from build123d import *

# Parameters (mm, degrees)
F1_DEPTH = 63.5
F2_DEPTH = 12.7
F3_R     = 5.08


with BuildPart() as f1:
    # F0 (on Front) → F1 (new body, symmetric)
    with BuildSketch(Plane.XZ):
        Polygon((19.77428763, 13.4614007547), (-32.80030936, 13.4614007547), (-32.80030936, -13.4614007547), (32.80030936, -13.4614007547), (32.80030936, 13.4614007547), align=None)
    extrude(amount=F1_DEPTH, both=True)

    # F0 (on Front) → F2 (join, symmetric)
    with BuildSketch(Plane.XZ):
        with BuildLine():
            Line((19.77428763, 24.8372294009), (19.77428763, 13.4614007547))
            Line((19.77428763, 13.4614007547), (32.80030936, 13.4614007547))
            Line((32.80030936, 13.4614007547), (32.80030936, 24.8372294009))
            ThreePointArc((32.80030936, 24.8372294009), (36.3320089212, 33.5525140508), (44.9345260859, 37.3506434262))
            Line((44.9345260859, 37.3506434262), (50.2432473004, 37.5140286498))
            Line((50.2432473004, 37.5140286498), (50.2432473004, 50.5462181007))
            Line((50.2432473004, 50.5462181007), (44.533817111, 50.3705003543))
            ThreePointArc((44.533817111, 50.3705003543), (26.9806216999, 42.6205237084), (19.77428763, 24.8372294009))
        make_face()
        Polygon((59.8447506625, 37.809531787), (50.2432473004, 37.5140286498), (50.2432473004, 33.1795029342), (59.9276782147, 33.1795029342), align=None)
        Polygon((59.5269692399, 55.5519722402), (59.8447506625, 37.809531787), (59.9276782147, 33.1795029342), (68.8237734139, 33.1795029342), (68.8237734139, 55.5519722402), align=None)
        Polygon((50.2432473004, 55.5519722402), (50.2432473004, 50.5462181007), (50.2432473004, 37.5140286498), (59.8447506625, 37.809531787), (59.5269692399, 55.5519722402), align=None)
    extrude(amount=F2_DEPTH, both=True)

    # F3
    f3_edges = [f1.edges().sort_by_distance(p)[0] for p in [
        (0, -63.5, 13.461401),
        (-32.800309, -63.5, 0),
        (0, -63.5, -13.461401),
        (32.800309, -63.5, 0),
        (-32.800309, 63.5, 0),
        (0, 63.5, -13.461401),
        (32.800309, 63.5, 0),
        (0, 63.5, 13.461401),
    ]]
    fillet(f3_edges, radius=F3_R)


solid = f1.part
For this review, take the finished solid that the model builds, in its own axes (mm). A direction names the side the tool comes from. Round coordinates to 2 decimals unless told otherwise and drop trailing zeros. Loops run counter-clockwise (first coordinate to the right, second up) from the corner with the lowest first, then second, coordinate; pieces in that order, holes last. Notation, with made-up numbers: (87, 78.5) - (121, 78.5) arc R34 cw to (121, 113.5) - close; hole circle Ø11 at (51, 14). An arc over 180 degrees is marked (long way). Use one line per item in the form item = value.
1) Wall thickness on probe 1 along Z at (x, y) = (15.5, 39); probe 2 along X at (y, z) = (12.5, 21); probe 3 along Z at (x, y) = (52, -8.5): over which ranges is each line inside the solid? List them lowest first.
Solutions:
probe_1 = -13.46 to 13.46
probe_2 = 19.77 to 32.8
probe_3 = 33.18 to 55.55
2) We need section C-C on z = -0.5. Write out the cut boundary in (x, y), then the cut area to 3 significant figures.
Solutions:
outline = (-32.8, -58.42) arc R5.08 ccw to (-27.72, -63.5) - (27.72, -63.5) arc R5.08 ccw to (32.8, -58.42) - (32.8, 58.42) arc R5.08 ccw to (27.72, 63.5) - (-27.72, 63.5) arc R5.08 ccw to (-32.8, 58.42) - close
area = 8,310 mm2
3) Mouldability with a two-part tool opening along X and no side actions: class faces 3 (the face through (0, -1, 13.461)), 4 (the face through (19.774, 0, 19)), 5 (the face through (36.239, -0.178, 33.455)) as pulls with the +X half, pulls with the -X half, needs draft (parallel to the pull), parting line crosses it, or undercut.
Solutions:
face_3 = needs draft
face_4 = pulls with the -X half
face_5 = undercut
4) We need section B-B on y = 5.5. Write out the cut boundary in (x, z), then the cut area to 3 significant figures.
Solutions:
outline = (-32.8, -13.46) - (32.8, -13.46) - (32.8, 24.84) arc R12.52 cw to (44.93, 37.35) - (50.24, 37.51) - (50.24, 33.18) - (68.82, 33.18) - (68.82, 55.55) - (50.24, 55.55) - (50.24, 50.55) - (44.53, 50.37) arc R25.55 ccw to (19.77, 24.84) - (19.77, 13.46) - (-32.8, 13.46) - close
area = 2,780 mm2
5) Clearance check with flat-ended pins moving along their axes: P1, Ø6, axis at y = 49, z = -6, coming from the +X side; P2, Ø10, axis at x = -1, y = 18, coming from the +Z side; P3, Ø3, axis at x = -20, z = 16, coming from the +Y side; P4, Ø9.5, axis at x = 62.5, y = 6.5, coming from the -Z side. State where each tip first meets the part, or that it passes through.
Solutions:
P1 = 32.8
P2 = 13.46
P3 = through
P4 = 33.18
6) We need section A-A on x = -8.5. Write out the cut boundary in (y, z).
Solutions:
outline = (-63.5, -8.38) arc R5.08 ccw to (-58.42, -13.46) - (58.42, -13.46) arc R5.08 ccw to (63.5, -8.38) - (63.5, 8.38) arc R5.08 ccw to (58.42, 13.46) - (-58.42, 13.46) arc R5.08 ccw to (-63.5, 8.38) - close
7) We need section D-D on y = -50. Write out the cut boundary in (x, z).
Solutions:
outline = (-32.8, -13.46) - (32.8, -13.46) - (32.8, 13.46) - (-32.8, 13.46) - close
8) Tool access review of faces 1 (the face through (0, -1, -13.461)), 2 (the face through (59, 0, 33.18)): name each direction out of +Z, -Z, +X, -X, +Y, -Y from which nothing blocks a thin tool from reaching the whole face with its end or side.
Solutions:
face_1 = -Z, +X, -X, +Y, -Y
face_2 = -Z, +X, +Y, -Y
